The drawing under review shows one solid part. Ordinate dimensions are in mm from its lowest x, y, z. A direction names the side the tool comes from. Give positions to 0.01 mm unless a question says otherwise; leave off trailing zeros. Write each loop counter-clockwise with the first axis right and the second up, starting at its lowest first coordinate (ties: lowest second). Pieces come first, ordered by that corner, then holes. Notation, with made-up numbers: M 70.5,78 L 75.5,78 A24 cw 75.5,99 Z; hole C -19,21.25 d6. An arc over 180 degrees is marked long. Answer as a JSON object with one key per item and string values. Group by question number.
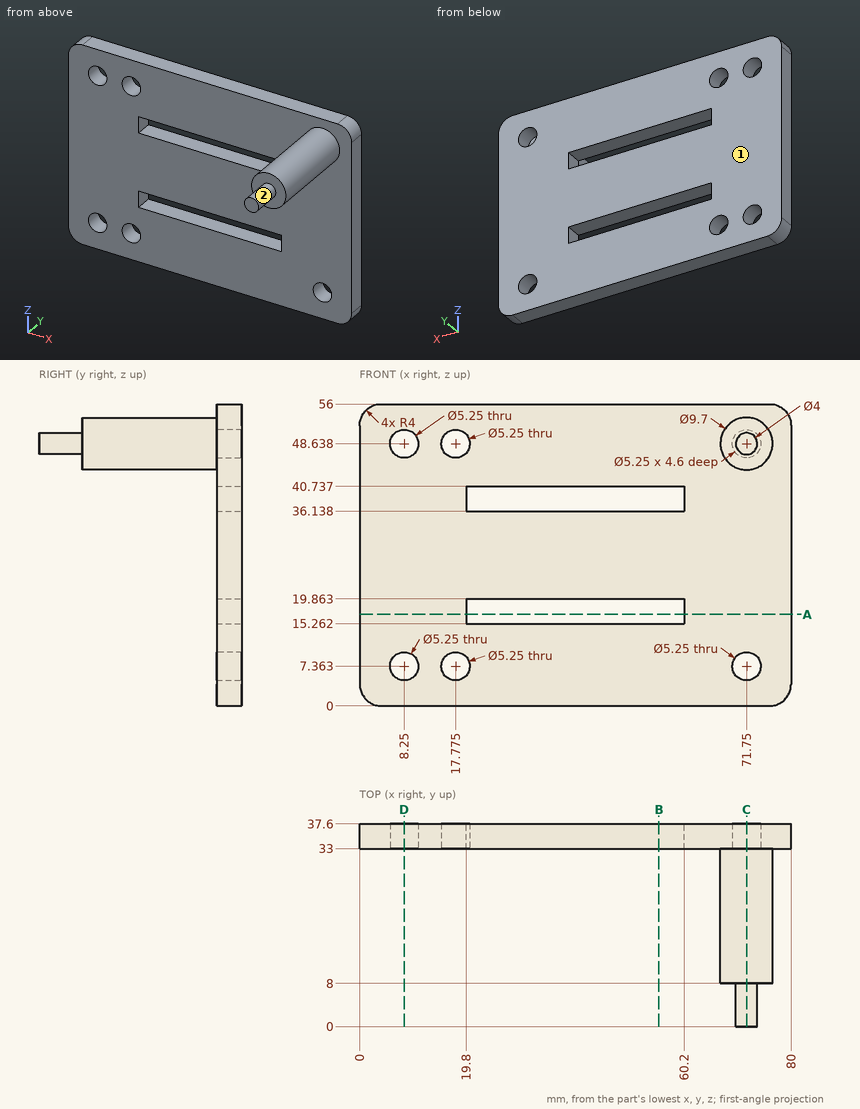
Item 1: Machinability: for the marked faces 1 and 2, which of the approach directions +Z, -Z, +X, -X, +Y, -Y give a long, thin tool a straight path to every point of the face, cutting with its end or side? Answer none if there is none.
Item 2: Consider section C-C (x = 71.75). Give the boundary of the cut face in (y, z).
Item 3: Insertion check: P1, Ø3, axis at x = 59.5, z = 23.5, coming from the -Y side. The pin has a flat end and moves straight along its axis. Give the tip position at first contact, or say it passes through.
Item 4: Consider section A-A (z = 17). Give the boundary of the cut face in (x, y).
Item 5: To check wall thickness, follow probe 1 along Z at (x, y) = (8.25, 34.2); probe 2 along Z at (x, y) = (71, 36); probe 3 along Y at (x, z) = (71.5, 10.5). State the ranges of each line that lie inside material, in increasing order.
Item 6: Consider section B-B (x = 55.5). Give the boundary of the cut face in (y, z).
Item 7: Consider section D-D (x = 8.25). Give the boundary of the cut face in (y, z).
Result set:
{
 "1": {"face 1": "+Z, -Z, +X, -X, +Y", "face 2": "-Y"},
 "2": {"outline": "M 0,46.64 L 8,46.64 L 8,43.79 L 33,43.79 L 33,9.99 L 37.6,9.99 L 37.6,46.01 L 33,46.01 L 33,51.26 L 37.6,51.26 L 37.6,56 L 33,56 L 33,53.49 L 8,53.49 L 8,50.64 L 0,50.64 Z; M 33,0 L 37.6,0 L 37.6,4.74 L 33,4.74 Z"},
 "3": {"P1": "stops at y = 33"},
 "4": {"outline": "M 0,33 L 19.8,33 L 19.8,37.6 L 0,37.6 Z; M 60.2,33 L 80,33 L 80,37.6 L 60.2,37.6 Z"},
 "5": {"probe 1": "z = 0 to 4.74, 9.99 to 46.01, 51.26 to 56", "probe 2": "z = 0 to 4.85, 9.88 to 46.12, 51.15 to 56", "probe 3": "y = 33 to 37.6"},
 "6": {"outline": "M 33,0 L 37.6,0 L 37.6,15.26 L 33,15.26 Z; M 33,19.86 L 37.6,19.86 L 37.6,36.14 L 33,36.14 Z; M 33,40.74 L 37.6,40.74 L 37.6,56 L 33,56 Z"},
 "7": {"outline": "M 33,0 L 37.6,0 L 37.6,4.74 L 33,4.74 Z; M 33,9.99 L 37.6,9.99 L 37.6,46.01 L 33,46.01 Z; M 33,51.26 L 37.6,51.26 L 37.6,56 L 33,56 Z"}
}
